Build history of the part. All positions in model axes, mm. A direction names the side the tool comes from. Round coordinates to 2 decimals unless told otherwise and drop trailing zeros. Write each loop counter-clockwise with the first axis right and the second up, starting at its lowest first coordinate (ties: lowest second). Pieces come first, ordered by that corner, then holes. Notation, with made-up numbers: (-17, 9) - (-11, 9) arc R13 ccw to (-11, 28) - close; hole circle Ø5 at (72.25, 80.5). An arc over 180 degrees is marked (long way). Write each question's results on one line, items separated by ' | '.
from build123d import *

# Parameters (mm, degrees)
F0_W     = 33
F0_H     = 12
F1_DEPTH = 3
F2_W     = 3
F2_H     = 9
F3_DEPTH = 17
F4_R     = 2
F5_DEPTH = 2
F6_SIZE  = 2


with BuildPart() as f1:
    # F0 (on Top) → F1 (new body)
    with BuildSketch(Plane.XY):
        Rectangle(F0_W, F0_H)
    extrude(amount=F1_DEPTH)

    # F2 (on face) → F3 (join)
    with BuildSketch(Plane.XY.offset(3)):
        with Locations((15, -1.5)):
            Rectangle(F2_W, F2_H)
    extrude(amount=F3_DEPTH)

    # F4 (on face) → F5 (cut)
    with BuildSketch(Plane(origin=(13.5, 0, 0), x_dir=(0, -1, 0), z_dir=(-1, 0, 0))):
        with Locations((1.5, 15.5)):
            Circle(F4_R)
    extrude(amount=-F5_DEPTH, mode=Mode.SUBTRACT)

    # F6
    f6_edges = [f1.edges().sort_by_distance(p)[0] for p in [
        (13.5, -1.5, 20),
    ]]
    chamfer(f6_edges, length=F6_SIZE)

    # F7: F1 across plane


with BuildPart() as f1_1:
    add(f1.part)
    add(f1.part.mirror(Plane.YZ))


solid = f1_1.part
(1) Two-plate mould, pull along Z, no slides. Class faces 1 (the flat face through (-16, -1, 20)), 2 (the flat face through (15.5, -1, 16)), 3 (the flat face through (-15, 3, 11)): released by +Z, released by -Z, zero draft, split by the parting line, or undercut.
Worked answers:
face 1: released by +Z | face 2: undercut | face 3: zero draft
(2) Tool access for faces 4 (the flat face through (15, 3, 11)), 5 (the cylindrical face through (-14.486, -1.24, 17.483)), 6 (the flat face through (14.5, -1.6, 19)): list every direction of +Z, -Z, +X, -X, +Y, -Y with a clear straight run to the whole face (end or side of a thin tool).
Worked answers:
face 4: +Z, +X, -X, +Y | face 5: none | face 6: +Z, +Y, -Y
(3) Drill centre lines: probe 1 along X at (y, z) = (-1.5, 6.5); probe 2 along Z at (x, y) = (1.5, 1.25); probe 3 along X at (y, z) = (-1.75, 15). Where is each one in solid material? Low to high. Write a range as [from, to].
Worked answers:
probe 1: x = [-16.5, -13.5], [13.5, 16.5] | probe 2: z = [0, 3] | probe 3: x = [-16.5, -15.5], [15.5, 16.5]
(4) Slice it at D-D, the plane x = -10. Write the cut outline in (y, z), and give its area (3 significant figures).
Worked answers:
outline: (-6, 0) - (6, 0) - (6, 3) - (-6, 3) - close | area: 36.0 mm2
(5) Slice it at B-B, the plane y = 2. Write the cut outline in (x, z), and give its area (3 significant figures).
Worked answers:
outline: (-16.5, 0) - (16.5, 0) - (16.5, 20) - (15.5, 20) - (13.5, 18) - (13.5, 3) - (-13.5, 3) - (-13.5, 18) - (-15.5, 20) - (-16.5, 20) - close | area: 197 mm2
(6) Slice it at C-C, the plane z = 16. Write the cut outline in (x, y).
Worked answers:
outline: (-16.5, -6) - (-13.5, -6) - (-13.5, -3.44) - (-15.5, -3.44) - (-15.5, 0.44) - (-13.5, 0.44) - (-13.5, 3) - (-16.5, 3) - close; (13.5, -6) - (16.5, -6) - (16.5, 3) - (13.5, 3) - (13.5, 0.44) - (15.5, 0.44) - (15.5, -3.44) - (13.5, -3.44) - close
(7) Flat gauge pins, fed straight in: pin 1 Ø0.9 at (x, z) = (-14.5, 12.5) entering from +Y; pin 2 Ø1.5 at (x, z) = (-12.5, 10.5) entering from +Y. Where does each tip first touch, or does it go through?
Worked answers:
pin 1: stops at y = 3 | pin 2: passes through
(8) Slice it at A-A, the plane z = 11.25. Write the cut outline in (x, y).
Worked answers:
outline: (-16.5, -6) - (-13.5, -6) - (-13.5, 3) - (-16.5, 3) - close; (13.5, -6) - (16.5, -6) - (16.5, 3) - (13.5, 3) - close
